from build123d import *

# Parameters (mm, degrees)
BASEHEAD_DEPTH  = 3.5
THDSCHPAT_COUNT = 12
THDSCHPAT_PITCH = 0.75


with BuildPart() as part:
    # Sketch1 → BaseHead (new body)
    with BuildSketch(Plane(origin=(0, 0, 0), x_dir=(0, 0, -1), z_dir=(1, 0, 0))):
        Polygon((4, 2.309401077), (4, -2.309401077), (0, -4.618802154), (-4, -2.309401077), (-4, 2.309401077), (0, 4.618802154), align=None)
    extrude(amount=BASEHEAD_DEPTH)

    # BodySke → BaseBody (revolve)
    with BuildSketch(Plane.XY):
        Polygon((0, 0), (18.5, 0), (18.5, 2.055), (18.055, 2.5), (0, 2.5), align=None)
    revolve(axis=Axis((0, 0, 0), (1, 0, 0)))

    # Sketch3 → HeadChamfer (revolve, cut)
    with BuildSketch(Plane.XY):
        Polygon((0, 4), (3.244016936, 9.618802154), (3.244016936, 14.618802154), (-10, 14.618802154), (-10, 4), align=None)
    revolve(axis=Axis((0, 0, 0), (1, 0, 0)), mode=Mode.SUBTRACT)

    # ThdSchSke → ThreadSchematic (revolve, cut)
    with BuildSketch(Plane.XY):
        Polygon((9.5, -2.055), (9.188407645, -2.5), (9.188407645, -3.125), (9.811592355, -3.125), (9.811592355, -2.5), align=None)
    threadschematic = revolve(axis=Axis((-3.175, 0, 0), (1, 0, 0)), mode=Mode.SUBTRACT)

    # ThdSchPat: ThreadSchematic ×12
    with Locations(*[(i * THDSCHPAT_PITCH, 0, 0) for i in range(1, THDSCHPAT_COUNT)]):
        add(threadschematic, mode=Mode.SUBTRACT)


solid = part.part
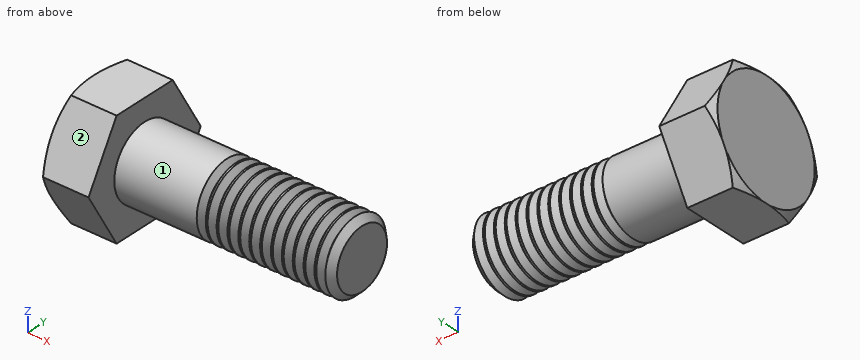
Work out the finished part from the listing and answer in its coordinate system (mm). Face numbers are marked on the shaded views. A direction names the side the tool comes from. Coordinates: 2 decimals unless noted, no trailing zeros. Answer as CSV lines item,"result".
1) Flat-ended cylindrical pins translate along their axes: pin 1 (1.5 mm diameter, centred on y = 3.5, z = -2, fed in from +X); pin 2 (1.5 mm diameter, centred on y = 2.5, z = 2, fed in from +X); pin 3 (2 mm diameter, centred on x = 11.5, y = 2.5, fed in from -Z). Find the tip coordinate at first contact, or state that the pin passes through.
A:
pin 1,"stops at x = 3.5"
pin 2,"stops at x = 18.1"
pin 3,"stops at z = -2"
2) The part is cut by section A-A (z = -2.25). State how many separate pieces and enclosed holes the cut face has, and give its area (3 significant figures).
A:
separate pieces,"13"
enclosed holes,"0"
area,"45.1 mm²"
3) Straight lines are drawn through the part: probe 1 along Z at (x, y) = (4.5, -1.5); probe 2 along X at (y, z) = (2.75, -0.5); probe 3 along Y at (x, z) = (15.25, -0.25). For each, find the intervals that lie inside material, in ascending order.
A:
probe 1,"z = -2 to 2"
probe 2,"x = 0 to 3.5"
probe 3,"y = -2.4 to 2.4"
4) For the marked faces 1 and 2, determine the directions among +Z, -Z, +X, -X, +Y, -Y from which every point of the face is accessible in a straight line to the end or side of a thin tool.
A:
face 1,"+X"
face 2,"+Z, +X, -X, -Y"
